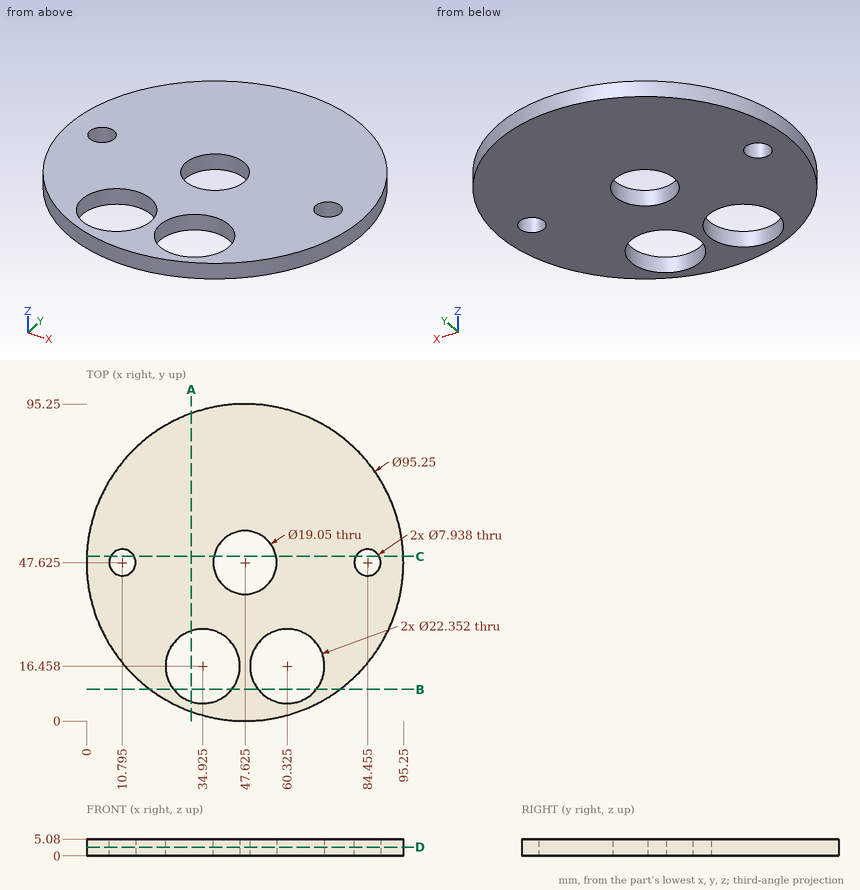
Print and shaded views of the part. All mm, measured from the part's lowest x, y and z. Round coordinates to 2 decimals unless told otherwise and drop trailing zeros. Order: outer loops, then holes, each group sorted by start corner. A loop starts at its lowest first (then second) coordinate and runs counter-clockwise, first axis right, second up. Notation, with made-up numbers: (25, 30) - (78, 30) arc R17 cw to (78, 42) - close; hole circle Ø2 at (27, -35.5). An arc over 180 degrees is marked (long way). Use a Markdown table: item, result.
1) Flat gauge pins, fed straight in: pin 1 Ø15 at (x, y) = (47.625, 47.625) entering from -Z; pin 2 Ø1.5 at (y, z) = (82.5, 2) entering from -X (1 decimal); pin 3 Ø1.5 at (x, z) = (61.5, 2.5) entering from -Y (1 decimal); pin 4 Ø1 at (y, z) = (74.5, 2) entering from +X. Where does each tip first touch, or does it go through?
Recorded:
| item | result |
|---|---|
| pin 1 | passes through |
| pin 2 | stops at x = 14.4 |
| pin 3 | stops at y = 1.8 |
| pin 4 | stops at x = 87.28 |
2) Saw through at B-B on y = 9.5. Write the cut outline in (x, z).
Recorded:
| item | result |
|---|---|
| outline | (19.08, 0) - (26.18, 0) - (26.18, 5.08) - (19.08, 5.08) - close; (43.67, 0) - (51.58, 0) - (51.58, 5.08) - (43.67, 5.08) - close; (69.07, 0) - (76.17, 0) - (76.17, 5.08) - (69.07, 5.08) - close |
3) Saw through at D-D on z = 2.65. Give the number of separate pieces and of enclosed holes in the cut face, and give its area (3 significant figures).
Recorded:
| item | result |
|---|---|
| separate pieces | 1 |
| enclosed holes | 5 |
| area | 5,960 mm² |
4) Saw through at C-C on y = 49.5. Write the cut outline in (x, z).
Recorded:
| item | result |
|---|---|
| outline | (0.04, 0) - (7.3, 0) - (7.3, 5.08) - (0.04, 5.08) - close; (14.29, 0) - (38.29, 0) - (38.29, 5.08) - (14.29, 5.08) - close; (56.96, 0) - (80.96, 0) - (80.96, 5.08) - (56.96, 5.08) - close; (87.95, 0) - (95.21, 0) - (95.21, 5.08) - (87.95, 5.08) - close |
5) Wall check: L1, parallel to Y at x = 42, z = 4.6 (1 decimal); L2, parallel to X at y = 48.5, z = 3.15 (1 decimal); L3, parallel to X at y = 22.5, z = 2.3 (1 decimal). Give the ranges that are in metal, low to high.
Recorded:
| item | result |
|---|---|
| L1 | y = 0.3 to 7.8, 25.1 to 39.9, 55.3 to 94.9 |
| L2 | x = 0 to 6.9, 14.7 to 38.1, 57.1 to 80.6, 88.3 to 95.2 |
| L3 | x = 7.2 to 25.5, 44.3 to 50.9, 69.7 to 88.1 |
6) Saw through at A-A on x = 31.5. Write the cut outline in (y, z), and give its area (3 significant figures).
Recorded:
| item | result |
|---|---|
| outline | (2.81, 0) - (5.82, 0) - (5.82, 5.08) - (2.81, 5.08) - close; (27.1, 0) - (92.44, 0) - (92.44, 5.08) - (27.1, 5.08) - close |
| area | 347 mm² |
